```python
from build123d import *

# Parameters (mm, degrees)
F0_W     = 69.85
F0_H     = 38.1
F1_DEPTH = 25.4
F2_R     = 6.35
F3_DEPTH = 25.4
F5_DEPTH = 12.7


with BuildPart() as f1:
    # F0 (on Front) → F1 (new body)
    with BuildSketch(Plane.XZ):
        with Locations((34.925, 19.05)):
            Rectangle(F0_W, F0_H)
    extrude(amount=F1_DEPTH)

    # F2 (on face) → F3 (cut)
    with BuildSketch(Plane.XZ.offset(25.4)):
        with Locations((12.7, 25.4)):
            Circle(F2_R)
        with BuildLine():
            ThreePointArc((12.7, 38.1), (21.680256, 34.380256), (25.4, 25.4))
            Line((25.4, 25.4), (25.4, 12.7))
            Line((25.4, 12.7), (69.85, 12.7))
            Line((69.85, 12.7), (69.85, 38.1))
            Line((69.85, 38.1), (12.7, 38.1))
        make_face()
        with BuildLine():
            ThreePointArc((0, 25.4), (3.719744, 34.380256), (12.7, 38.1))
            Line((12.7, 38.1), (0, 38.1))
            Line((0, 38.1), (0, 25.4))
        make_face()
    extrude(amount=-F3_DEPTH, mode=Mode.SUBTRACT)

    # F4 (on face) → F5 (cut)
    with BuildSketch(Plane.XY.offset(12.7)):
        with BuildLine():
            ThreePointArc((57.15, -19.05), (50.8, -12.7), (57.15, -6.35))
            Line((57.15, -6.35), (38.1, -6.35))
            ThreePointArc((38.1, -6.35), (42.590128, -8.209872), (44.45, -12.7))
            ThreePointArc((44.45, -12.7), (42.590128, -17.190128), (38.1, -19.05))
            Line((38.1, -19.05), (57.15, -19.05))
        make_face()
        with BuildLine():
            ThreePointArc((44.45, -12.7), (42.590128, -8.209872), (38.1, -6.35))
            ThreePointArc((38.1, -6.35), (31.75, -12.7), (38.1, -19.05))
            ThreePointArc((38.1, -19.05), (42.590128, -17.190128), (44.45, -12.7))
        make_face()
        with BuildLine():
            ThreePointArc((57.15, -19.05), (61.640128, -17.190128), (63.5, -12.7))
            ThreePointArc((63.5, -12.7), (61.640128, -8.209872), (57.15, -6.35))
            ThreePointArc((57.15, -6.35), (50.8, -12.7), (57.15, -19.05))
        make_face()
    extrude(amount=-F5_DEPTH, mode=Mode.SUBTRACT)


solid = f1.part
```
For this review, take the finished solid that the model builds, in its own axes (mm). A direction names the side the tool comes from. Round coordinates to 2 decimals unless told otherwise and drop trailing zeros. Loops run counter-clockwise (first coordinate to the right, second up) from the corner with the lowest first, then second, coordinate; pieces in that order, holes last.
(1) We need section A-A (x = 55.5). Give the boundary of the cut face in (y, z), plus the area to 3 significant figures.
Returned:
outline: (-25.4, 0) - (-19.05, 0) - (-19.05, 12.7) - (-25.4, 12.7) - close; (-6.35, 0) - (0, 0) - (0, 12.7) - (-6.35, 12.7) - close
area: 161 mm2
(2) We need section B-B (y = -13.5). Give the boundary of the cut face in (x, z), plus the area to 3 significant figures.
Returned:
outline: (0, 0) - (31.8, 0) - (31.8, 12.7) - (25.4, 12.7) - (25.4, 25.4) arc R12.7 ccw to (0, 25.4) - close; (63.45, 0) - (69.85, 0) - (69.85, 12.7) - (63.45, 12.7) - close; hole circle Ø12.7 at (12.7, 25.4)
area: 934 mm2
(3) Wall thickness on line 1 along Z through (x, y) = (12.7, -16.25); line 2 along Y through (x, z) = (44.5, 7); line 3 along Z through (x, y) = (40.5, -1.25): over which ranges is each line inside the solid? List them lowest first.
Returned:
line 1: z = 0 to 19.05, 31.75 to 38.1
line 2: y = -25.4 to -19.05, -6.35 to 0
line 3: z = 0 to 12.7
(4) Tool access review of faces 5 (the flat face through (69.85, -13, 6)), 6 (the flat face through (47, -21, 12.7)), 7 (the flat face through (48, -6.35, 6)): name each direction out of +Z, -Z, +X, -X, +Y, -Y from which nothing blocks a thin tool from reaching the whole face with its end or side.
Returned:
face 5: +Z, -Z, +X, +Y, -Y
face 6: +Z, +X, +Y, -Y
face 7: +Z, -Z
(5) Mouldability with a two-part tool opening along X and no side actions: class faces 1 (the flat face through (27, -25.4, 11)), 2 (the cylindrical face through (31.75, -12.56, 6.44)), 3 (the flat face through (25.4, -13, 19)), 4 (the flat face through (0, -13, 13)) as released by +X, released by -X, zero draft, split by the parting line, or undercut.
Returned:
face 1: zero draft
face 2: undercut
face 3: released by +X
face 4: released by -X
(6) We need section C-C (z = 12). Give the boundary of the cut face in (x, y).
Returned:
outline: (0, -25.4) - (69.85, -25.4) - (69.85, 0) - (0, 0) - close; hole (38.1, -19.05) - (57.15, -19.05) arc R6.35 ccw to (57.15, -6.35) - (38.1, -6.35) arc R6.35 ccw to start
(7) We need section D-D (y = -4.75). Give the boundary of the cut face in (x, z).
Returned:
outline: (0, 0) - (69.85, 0) - (69.85, 12.7) - (25.4, 12.7) - (25.4, 25.4) arc R12.7 ccw to (0, 25.4) - close; hole circle Ø12.7 at (12.7, 25.4)
(8) Clearance check with flat-ended pins moving along their axes: P1, Ø3, axis at x = 20.5, y = -7, coming from the +Z side; P2, Ø12, axis at y = -17, z = 23.5, coming from the +X side; P3, Ø7.5, axis at x = 46, y = -14, coming from the +Z side. State where each tip first meets the part, or that it passes through.
Returned:
P1: stops at z = 36.43
P2: stops at x = 25.4
P3: passes through
